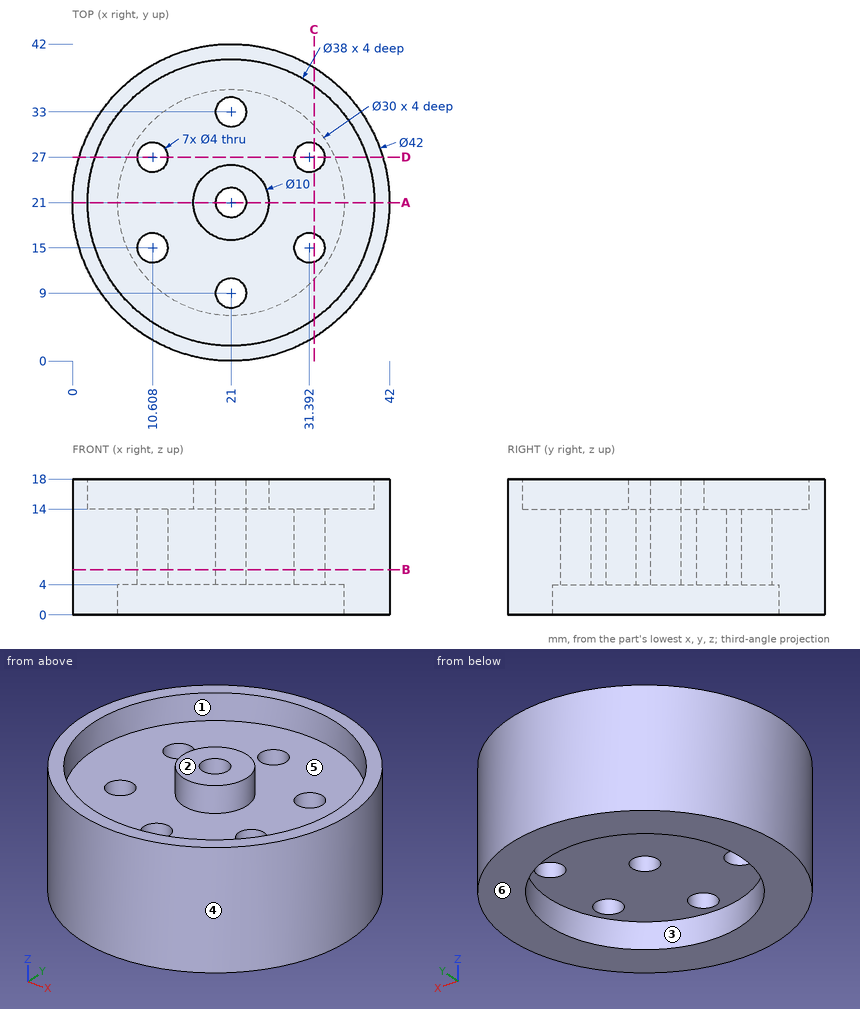
Geometry: see drawing. Coordinates: mm, zero at the bounding-box minimum. A direction names the side the tool comes from. Coordinates: 2 decimals unless noted, no trailing zeros. Loops run counter-clockwise (first coordinate to the right, second up) from the corner with the lowest first, then second, coordinate; pieces in that order, holes last. Notation, with made-up numbers: (37.25, 24.25) -> (95.25, 24.25) arc R16 cw to (95.25, 52.25) -> close; hole circle Ø10 at (77.5, -11). An arc over 180 degrees is marked (long way). Write item = value, one per line. Start each with the question number.
Item 1: Reachability of the marked faces 1, 2 and 3 from +Z, -Z, +X, -X, +Y, -Y: full face, straight path, thin tool, end or side. Return the list, or none.
Item 2: Cut plane D-D, the plane y = 27. Return loops of the section in (x, z) (1 decimal).
Item 3: Cut plane A-A, the plane y = 21. Return loops of the section in (x, z), plus the area to 3 significant figures.
Item 4: Cut plane C-C, the plane x = 32. Return loops of the section in (y, z) (1 decimal), plus the area to 3 significant figures.
Item 5: Material intervals for line 1 (Y direction, x = 25, z = 16) (1 decimal); line 2 (X direction, y = 20.5, z = 1.75); line 3 (Y direction, x = 10, z = 9.5) (1 decimal), sorted ascending.
Item 6: First-contact query: P1, Ø15, axis at x = 27.5, y = 24, coming from the -Z side; P2, Ø10, axis at x = 33.5, z = 12.5, coming from the -Y side (1 decimal); P3, Ø1, axis at x = 17, z = 12.5, coming from the +Y side; P4, Ø6.5, axis at x = 31.39, y = 15, coming from the -Z side. Flat tips, straight axial feed; report the tip coordinate or a pass-through.
Item 7: Cut plane B-B, the plane z = 6. Return loops of the section in (x, y).
Item 8: Mould query, pull axis X, two halves, no side actions, for the marked faces 4, 5 and 6. Classes: pulls with the +X half, pulls with the -X half, needs draft (parallel to the pull), parting line crosses it, or undercut.
Ans:
q1.face_1 = +Z
q1.face_2 = +Z, +X, -X, +Y, -Y
q1.face_3 = -Z
q2.outline = (0.9, 0) -> (7.3, 0) -> (7.3, 4) -> (8.6, 4) -> (8.6, 14) -> (3, 14) -> (3, 18) -> (0.9, 18) -> close; (12.6, 4) -> (29.4, 4) -> (29.4, 14) -> (12.6, 14) -> close; (33.4, 4) -> (34.7, 4) -> (34.7, 0) -> (41.1, 0) -> (41.1, 18) -> (39, 18) -> (39, 14) -> (33.4, 14) -> close
q3.outline = (0, 0) -> (6, 0) -> (6, 4) -> (19, 4) -> (19, 18) -> (16, 18) -> (16, 14) -> (2, 14) -> (2, 18) -> (0, 18) -> close; (23, 4) -> (36, 4) -> (36, 0) -> (42, 0) -> (42, 18) -> (40, 18) -> (40, 14) -> (26, 14) -> (26, 18) -> (23, 18) -> close
q3.area = 468 mm²
q4.outline = (3.1, 0) -> (10.8, 0) -> (10.8, 4) -> (13.1, 4) -> (13.1, 14) -> (5.5, 14) -> (5.5, 18) -> (3.1, 18) -> close; (16.9, 4) -> (25.1, 4) -> (25.1, 14) -> (16.9, 14) -> close; (28.9, 4) -> (31.2, 4) -> (31.2, 0) -> (38.9, 0) -> (38.9, 18) -> (36.5, 18) -> (36.5, 14) -> (28.9, 14) -> close
q4.area = 362 mm²
q5.line_1 = 0.4 to 2.4, 18 to 24, 39.6 to 41.6
q5.line_2 = 0.01 to 6.01, 35.99 to 41.99
q5.line_3 = 3.1 to 13.1, 16.9 to 25.1, 28.9 to 38.9
q6.P1 = 4
q6.P2 = 1.4
q6.P3 = 41.71
q6.P4 = 0
q7.outline = circle Ø42 at (21, 21); hole circle Ø4 at (10.61, 15); hole circle Ø4 at (10.61, 27); hole circle Ø4 at (21, 9); hole circle Ø4 at (21, 21); hole circle Ø4 at (21, 33); hole circle Ø4 at (31.39, 15); hole circle Ø4 at (31.39, 27)
q8.face_4 = parting line crosses it
q8.face_5 = undercut
q8.face_6 = needs draft
